```python
from build123d import *

# Parameters (mm, degrees)
EXTRUDE_THIN2_DEPTH = 476.25
FILLET1_R           = 1.016


with BuildPart() as part:
    # Sketch1 → Extrude-Thin2 (new body)
    with BuildSketch(Plane.XY):
        with BuildLine():
            Line((-6.35, 0), (-2.38125, 0))
            Line((-2.38125, 0), (-2.38125, 8.112125))
            Line((-2.38125, 8.112125), (-6.35, 10.0965))
            Line((-6.35, 10.0965), (-6.35, 17.24025))
            Line((-6.35, 17.24025), (-23.8125, 17.24025))
            Line((-23.8125, 17.24025), (-23.8125, 21.209))
            Line((-23.8125, 21.209), (-19.05, 21.209))
            Line((-19.05, 21.209), (-19.05, 23.59025))
            ThreePointArc((-19.05, 23.59025), (-15.568214533, 24.697581116), (-12.633740801, 26.874247409))
            ThreePointArc((-12.633740801, 26.874247409), (-8.42347359, 29.293600923), (-3.571875, 29.089609403))
            Line((-3.571875, 29.089609403), (-3.571875, 32.3215))
            Line((-3.571875, 32.3215), (3.571875, 32.3215))
            Line((3.571875, 32.3215), (3.571875, 29.089609403))
            ThreePointArc((3.571875, 29.089609403), (8.42347359, 29.293600923), (12.633740801, 26.874247409))
            ThreePointArc((12.633740801, 26.874247409), (15.568214533, 24.697581116), (19.05, 23.59025))
            Line((19.05, 23.59025), (19.05, 21.209))
            Line((19.05, 21.209), (23.8125, 21.209))
            Line((23.8125, 21.209), (23.8125, 17.24025))
            Line((23.8125, 17.24025), (6.35, 17.24025))
            Line((6.35, 17.24025), (6.35, 10.0965))
            Line((6.35, 10.0965), (2.38125, 8.112125))
            Line((2.38125, 8.112125), (2.38125, 0))
            Line((2.38125, 0), (6.35, 0))
            Line((6.35, 0), (6.35, -1.016))
            Line((6.35, -1.016), (1.36525, -1.016))
            Line((1.36525, -1.016), (1.36525, 8.740047533))
            Line((1.36525, 8.740047533), (5.334, 10.724422533))
            Line((5.334, 10.724422533), (5.334, 18.25625))
            Line((5.334, 18.25625), (22.7965, 18.25625))
            Line((22.7965, 18.25625), (22.7965, 20.193))
            Line((22.7965, 20.193), (18.034, 20.193))
            Line((18.034, 20.193), (18.034, 22.742528034))
            ThreePointArc((18.034, 22.742528034), (14.714811847, 24.002111564), (11.902541871, 26.168836802))
            ThreePointArc((11.902541871, 26.168836802), (7.461841431, 28.446841183), (2.555875, 27.529989099))
            Line((2.555875, 27.529989099), (2.555875, 31.3055))
            Line((2.555875, 31.3055), (-2.555875, 31.3055))
            Line((-2.555875, 31.3055), (-2.555875, 27.529989099))
            ThreePointArc((-2.555875, 27.529989099), (-7.461841431, 28.446841183), (-11.902541871, 26.168836802))
            ThreePointArc((-11.902541871, 26.168836802), (-14.714811847, 24.002111564), (-18.034, 22.742528034))
            Line((-18.034, 22.742528034), (-18.034, 20.193))
            Line((-18.034, 20.193), (-22.7965, 20.193))
            Line((-22.7965, 20.193), (-22.7965, 18.25625))
            Line((-22.7965, 18.25625), (-5.334, 18.25625))
            Line((-5.334, 18.25625), (-5.334, 10.724422533))
            Line((-5.334, 10.724422533), (-1.36525, 8.740047533))
            Line((-1.36525, 8.740047533), (-1.36525, -1.016))
            Line((-1.36525, -1.016), (-6.35, -1.016))
            Line((-6.35, -1.016), (-6.35, 0))
        make_face()
    extrude(amount=-EXTRUDE_THIN2_DEPTH)

    # Fillet1
    fillet1_edges = [part.edges().sort_by_distance(p)[0] for p in [
        (-6.35, 10.0965, -238.125),
        (-23.8125, 17.24025, -238.125),
        (-23.8125, 21.209, -238.125),
        (-19.05, 23.59025, -238.125),
        (-3.571875, 32.3215, -238.125),
        (3.571875, 32.3215, -238.125),
        (19.05, 23.59025, -238.125),
        (23.8125, 21.209, -238.125),
        (23.8125, 17.24025, -238.125),
        (6.35, 10.0965, -238.125),
        (1.36525, -1.016, -238.125),
        (1.36525, 8.740047533, -238.125),
        (5.334, 18.25625, -238.125),
        (18.034, 20.193, -238.125),
        (2.555875, 27.529989099, -238.125),
        (-2.555875, 27.529989099, -238.125),
        (-18.034, 20.193, -238.125),
        (-5.334, 18.25625, -238.125),
        (-1.36525, 8.740047533, -238.125),
        (-1.36525, -1.016, -238.125),
    ]]
    fillet(fillet1_edges, radius=FILLET1_R)


solid = part.part
```
Could you check a few things on this model? Use its own coordinates, in mm. A direction names the side the tool comes from. Coordinates: 2 decimals unless noted, no trailing zeros. Put each result on its own line as item: value. Start each with the question number.
(1) I need wall thicknesses on line 1 (X direction, y = 5, z = -108.5); line 2 (X direction, y = 22, z = -364.5); line 3 (Y direction, x = 7.5, z = -132.5). Which ranges of each line are inside material? Lowest first, please. Write a range as from..to.
(2) For faces 1 (the face through (2.381, 4, -235)), 2 (the face through (15, 17.24, -235)), 3 (the face through (8.241, 28.292, -234.791)), 4 (the face through (-1.365, 4, -235)), 5 (the face through (7, 18, -476.25)), which set-ups out of +Z, -Z, +X, -X, +Y, -Y let a thin tool reach every point of the face, with its end or its side?
(3) Thinking about a two-plate mould opening in X: for faces 6 (the face through (-14, 17.24, -235)), 7 (the face through (-2.381, 4, -235)), 8 (the face through (14, 18.256, -235)), which applies, pulls with the +X half, pulls with the -X half, needs draft (parallel to the pull), parting line crosses it, or undercut?
(4) Will these pins go through, and if not, where does the flat tip stop? P1, Ø7, axis at y = 13.5, z = -159.5, coming from the +X side; P2, Ø6, axis at y = 6, z = -300, coming from the -X side; P3, Ø2.5, axis at y = 3, z = -241.5, coming from the +X side.
Solutions:
1. line 1: x = -2.38..-1.37, 1.37..2.38
1. line 2: x = -19.05..-18.03, 18.03..19.05
1. line 3: y = 17.24..18.26, 28.44..29.47
2. face 1: +Z, -Z, +X
2. face 2: +Z, -Z, +X, -Y
2. face 3: +Z, -Z
2. face 4: +Z, -Z, -Y
2. face 5: -Z, +X, -X, +Y, -Y
3. face 6: needs draft
3. face 7: pulls with the -X half
3. face 8: undercut
4. P1: stops at x = 6.35
4. P2: stops at x = -4.16
4. P3: stops at x = 2.38
